Read the model definition and answer for the solid it produces. Units are mm, in the model's axes. Coordinates: 2 decimals unless noted, no trailing zeros. Write each loop counter-clockwise with the first axis right and the second up, starting at its lowest first coordinate (ties: lowest second). Pieces come first, ordered by that corner, then holes.
(1) Determine the mould class of faces 1 (the flat face through (-54, 49, 0)), 2 (the cylindrical face through (-67.69, 24.16, -14.25)), 3 (the cylindrical face through (-19.39, 24.16, -11.54)) for opening direction Z: pulls with the +Z half, pulls with the -Z half, needs draft (parallel to the pull), parting line crosses it, or undercut.
(2) The part is cut by section B-B, the plane z = 3.75. Determine the outline of the cut face in (x, y), and give its area (3 significant figures).
(3) Straight lines are drawn through the part: line 1 along X through (y, z) = (4.5, 6.75); line 2 along Z through (x, y) = (-46, 39.5); line 3 along Z through (x, y) = (-39.5, 42). For each, find the intervals that lie inside material, in ascending order.
(4) The part is cut by section A-A, the plane z = 11.75. Determine the outline of the cut face in (x, y), and give its area (3 significant figures).
(5) Given pin 1 (1 mm diameter, centred on x = -34.5, y = 10, fed in from +Z); pin 2 (5 mm diameter, centred on y = 23, z = -4, fed in from -X); pin 3 (6 mm diameter, centred on x = -46.5, y = 37, fed in from +Z), each flat-ended and moving along its own axis, determine where each tip first touches the part or whether it passes through.
```python
from build123d import *

# Parameters (mm, degrees)
BOSS_EXTRUDE1_DEPTH = 49
FILLET1_R           = 10
FILLET2_R           = 5


with BuildPart() as part:
    # Sketch1 → Boss-Extrude1 (new body)
    with BuildSketch(Plane(origin=(0, 0, 0), x_dir=(1, 0, 0), z_dir=(0, 1, 0))):
        with BuildLine():
            ThreePointArc((-74.859210096, 7.125), (-87.022345912, 12.163135816), (-81.984210096, 0))
            ThreePointArc((-81.984210096, 0), (-87.022345912, -12.163135816), (-74.859210096, -7.125))
            ThreePointArc((-74.859210096, -7.125), (-67.734210096, -14.25), (-60.609210096, -7.125))
            ThreePointArc((-60.609210096, -7.125), (-53.484210096, -14.25), (-46.359210096, -7.125))
            ThreePointArc((-46.359210096, -7.125), (-39.234210096, -14.25), (-32.109210096, -7.125))
            ThreePointArc((-32.109210096, -7.125), (-19.94607428, -12.163135816), (-24.984210096, 0))
            ThreePointArc((-24.984210096, 0), (-19.94607428, 12.163135816), (-32.109210096, 7.125))
            ThreePointArc((-32.109210096, 7.125), (-39.234210096, 14.25), (-46.359210096, 7.125))
            ThreePointArc((-46.359210096, 7.125), (-53.484210096, 14.25), (-60.609210096, 7.125))
            ThreePointArc((-60.609210096, 7.125), (-67.734210096, 14.25), (-74.859210096, 7.125))
        make_face()
    extrude(amount=BOSS_EXTRUDE1_DEPTH)

    # Fillet1
    fillet1_edges = [part.edges().sort_by_distance(p)[0] for p in [
        (-74.859210096, 24.5, -7.125),
        (-60.609210096, 24.5, -7.125),
        (-46.359210096, 24.5, -7.125),
        (-32.109210096, 24.5, -7.125),
        (-32.109210096, 24.5, 7.125),
        (-46.359210096, 24.5, 7.125),
        (-60.609210096, 24.5, 7.125),
        (-74.859210096, 24.5, 7.125),
    ]]
    fillet(fillet1_edges, radius=FILLET1_R)

    # Fillet2
    fillet2_edges = [part.edges().sort_by_distance(p)[0] for p in [
        (-81.984210096, 24.5, 0),
        (-24.984210096, 24.5, 0),
    ]]
    fillet(fillet2_edges, radius=FILLET2_R)


solid = part.part
```
Computed:
1. face 1: needs draft
1. face 2: pulls with the -Z half
1. face 3: undercut
2. outline: (-88.26, 0) - (-18.71, 0) - (-18.71, 49) - (-88.26, 49) - close
2. area: 3,410 mm2
3. line 1: x = -89.1 to -17.87
3. line 2: z = -12.7 to 12.7
3. line 3: z = -14.25 to 14.25
4. outline: (-87.4, 0) - (-19.56, 0) - (-19.56, 49) - (-87.4, 49) - close
4. area: 3,320 mm2
5. pin 1: stops at z = 13.12
5. pin 2: stops at x = -89.08
5. pin 3: stops at z = 13.2
